The model under review builds one solid part; all positions refer to its coordinate system, in mm. A direction names the side the tool comes from. Give positions to 0.01 mm unless a question says otherwise; leave off trailing zeros. Order: outer loops, then holes, each group sorted by start corner. A loop starts at its lowest first (then second) coordinate and runs counter-clockwise, first axis right, second up. Notation, with made-up numbers: (27, 65.25) - (72, 65.25) arc R21 ccw to (72, 69.25) - close; hole circle Ø10 at (15.25, 27.5). An arc over 180 degrees is marked (long way). Put each result on its own line as item: value.
Autodesk Inventor part; units mm, degrees
ref_plane "YZ Plane" through (0, 0, 0) normal (1, 0, 0) x (0, 1, 0)
ref_plane "XZ Plane" through (0, 0, 0) normal (0, 1, 0) x (-1, 0, 0)
ref_plane "XY Plane" through (0, 0, 0) normal (0, 0, 1) x (1, 0, 0)
sketch "Sketch1" plane through (0, 0, 0) normal (0, 1, 0) x (-1, 0, 0)
  line L0 (0, 0) -> (25.4, 0)
  line L1 (25.4, 0) -> (25.4, -25.4)
  line L2 (25.4, -25.4) -> (0, -25.4)
  line L3 (0, -25.4) -> (0, 0)
  line L4 (3.175, -3.175) -> (22.225, -3.175)
  line L5 (22.225, -3.175) -> (22.225, -22.225)
  line L6 (22.225, -22.225) -> (3.175, -22.225)
  line L7 (3.175, -22.225) -> (3.175, -3.175)
  dimension "d0" = 25.4
  dimension "d1" = 25.4
  dimension "d2" = 19.05
  dimension "d3" = 19.05
  dimension "d4" = 3.175
  dimension "d5" = 3.175
extrude "Extrusion1" add sketch "Sketch1" along normal blind 850.9
sketch "Sketch2" plane through (-25.4, 0, -25.4) normal (-1, 0, 0) x (0, 0, 1)
  line L0 (25.4, 0) -> (0, 0)
  line L1 (25.4, 0) -> (25.4, 850.9)
  line L2 (0, 850.9) -> (25.4, 850.9)
  line L3 (0, 0) -> (0, 850.9)
  point P0 (12.7, 812.8)
  point P1 (12.7, 787.4)
  point P2 (12.7, 12.7)
  point P3 (12.7, 38.1)
  dimension "d8" = 12.7
  dimension "d9" = 38.1
  dimension "d12" = 12.7
  dimension "d13" = 12.7
  dimension "d14" = 12.7
  dimension "d15" = 12.7
  dimension "d23" = 812.8
  dimension "d24" = 787.4
hole "Hole1" at (-25.4, 812.8, -12.7) at (-25.4, 787.4, -12.7) at (-25.4, 12.7, -12.7) at (-25.4, 38.1, -12.7) direction (1, 0, 0) diameter 3.9688 end through all
sketch "Sketch3" plane through (-25.4, 0, -25.4) normal (-1, 0, 0) x (0, 0, 1)
  circle A0 centre (12.7, 12.7) radius 1.9844
  circle A1 centre (12.7, 812.8) radius 1.9844
  circle A2 centre (12.7, 787.4) radius 1.9844
  circle A3 centre (12.7, 38.1) radius 1.9844
  line L0 (25.4, 0) -> (0, 0)
  line L1 (25.4, 0) -> (25.4, 850.9)
  line L2 (0, 850.9) -> (25.4, 850.9)
  line L3 (0, 0) -> (0, 850.9)
  line L4 (25.4, 850.9) -> (0, 850.9)
  line L5 (0, 850.9) -> (0, 812.8)
  line L6 (0, 0) -> (0, 850.9)
  line L7 (0, 812.8) -> (25.4, 850.9)
  dimension "d25" = 38.1
extrude "Extrusion2" cut sketch "Sketch3" against normal blind 25.4 contours L7 L3 L2
properties part number "1x1 support"
(1) Take a section at A-A, the plane y = 363. Write out the cut boundary in (x, z) (3 decimals).
The answers:
outline: (-25.4, -25.4) - (0, -25.4) - (0, 0) - (-25.4, 0) - close; hole (-22.225, -22.225) - (-3.175, -22.225) - (-3.175, -3.175) - (-22.225, -3.175) - close
(2) For faces 5 (the flat face through (-22.225, 417, -13)), 6 (the flat face through (-13, 419, 0)), list the 3-axis set-ups (+Z, -Z, +X, -X, +Y, -Y) from which the entire face can be reached by the end or side of a thin tool; tool diameter is ignored.
The answers:
face 5: +Y, -Y
face 6: +Z, +X, -X, +Y, -Y
(3) Clearance check with flat-ended pins moving along their axes: pin 1 Ø2.5 at (y, z) = (38.1, -12.7) entering from +X; pin 2 Ø4.5 at (y, z) = (787.4, -12.7) entering from -X. State where each tip first meets the part, or that it passes through.
The answers:
pin 1: through
pin 2: x = -25.4
(4) Wall thickness on L1, parallel to X at y = 430, z = -6.25 (3 decimals); L2, parallel to Z at x = -23.4, y = 38.1: over which ranges is each line inside the solid? List them lowest first.
The answers:
L1: -25.4 to -22.225, -3.175 to 0
L2: -25.4 to -14.68, -10.72 to 0
(5) Take a section at B-B, the plane x = -16. Write out the cut boundary in (y, z) (1 decimal).
The answers:
outline: (0, -25.4) - (812.8, -25.4) - (817.6, -22.2) - (0, -22.2) - close; (0, -3.2) - (846.1, -3.2) - (850.9, 0) - (0, 0) - close
(6) The part is to be moulded in two halves that separate along X. For faces 1 (the flat face through (-25.4, 419, -13)), 2 (the flat face through (0, 419, -13)), 3 (the flat face through (-13, 403, -22.225)), 4 (the flat face through (-13, 401, -25.4)), say which applies: pulls with the +X half, pulls with the -X half, needs draft (parallel to the pull), parting line crosses it, or undercut.
The answers:
face 1: pulls with the -X half
face 2: pulls with the +X half
face 3: undercut
face 4: needs draft
